Autodesk Inventor part; units mm, degrees
ref_plane "YZ Plane" through (0, 0, 0) normal (1, 0, 0) x (0, 1, 0)
ref_plane "XZ Plane" through (0, 0, 0) normal (0, 1, 0) x (-1, 0, 0)
ref_plane "XY Plane" through (0, 0, 0) normal (0, 0, 1) x (1, 0, 0)
sketch "스케치1" plane through (0, 0, 0) normal (0, 0, 1) x (1, 0, 0)
  line L0 (0, 0) -> (8.4524, -18.1262)
  line L1 (0, 0) -> (20, 0) construction
  line L2 (8.4524, -18.1262) -> (14.7965, -15.1678)
  line L3 (8.4524, -18.1262) -> (16.9047, -36.2523)
  line L4 (8.4524, -18.1262) -> (28.4524, -18.1262) construction
  arc A0 (16.9047, -36.2523) -> (0, 0) centre (-14.2701, -28.7218) ccw
  line L5 (0, 0) -> (0, 50)
  line L6 (0, 0) -> (50, 0) construction
  line L7 (0, 50) -> (12, 50)
  line L8 (12, 50) -> (12, 3)
  circle A1 centre (6, 44) radius 4.025
  circle A2 centre (6, 9) radius 4.025
  line L9 (16.9047, -36.2523) -> (26.8143, -31.6314)
  line L10 (16.9047, -36.2523) -> (27.8387, -36.2523) construction
  line L11 (12, -47.3039) -> (11.9482, -47.1928)
  arc A3 (26.2229, -36.2523) -> (12, 3) centre (-14.2701, -28.7218) ccw
  dimension "d16" = 20
  dimension "d17" = 65
  dimension "d18" = 7
  dimension "d19" = 90
  dimension "d20" = 20
  dimension "d21" = 65
  dimension "d22" = 50
  dimension "d23" = 90
  dimension "d24" = 12
  dimension "d25" = 90
  dimension "d26" = 47
  dimension "d27" = 8.05
  dimension "d28" = 8.05
  dimension "d29" = 6
  dimension "d30" = 6
  dimension "d31" = 6
  dimension "d32" = 35
  dimension "d33" = 25
extrude "돌출1" add sketch "스케치1" along normal blind 4 contours L5 L7 L8 A3 L9 A0
fillet "모깎기1" radius 6 2 edges at (12, 50, 2) (0, 50, 2)
sketch "스케치2" plane through (0, 0, 4) normal (0, 0, 1) x (1, 0, 0)
  line L0 (16.9047, -36.2523) -> (26.8143, -31.6314)
  arc A0 (17.3077, -34.3271) -> (18.715, -35.4082) centre (18.2923, -34.5019) ccw
  arc A1 (26.2765, -31.8822) -> (26.8523, -31.032) centre (25.8539, -30.9759) ccw
  line L1 (20, -34.809) -> (17.8869, -30.2774)
  line L2 (20, -34.809) -> (25, -34.809) construction
  line L3 (17.8869, -30.2774) -> (26.834, -26.1053)
  arc A2 (26.8143, -31.6314) -> (12, 3) centre (-14.2701, -28.7218) ccw
  line L4 (26.834, -26.1053) -> (17.7607, -30.3363)
  arc A3 (16.9047, -36.2523) -> (0, 0) centre (-14.2701, -28.7218) ccw
  arc A4 (26.2765, -31.8822) -> (26.8523, -31.032) centre (25.8539, -30.9759) ccw
  line L5 (26.834, -26.1053) -> (16.9047, -36.2523)
  line L6 (17.7607, -30.3363) -> (26.8143, -31.6314)
  circle A5 centre (22.0881, -30.9553) radius 1.6
  point P0 (12.3536, 2.7038)
  point P1 (0.5383, -0.2738)
  dimension "d38" = 5
  dimension "d39" = 115
  dimension "d40" = 90
  dimension "d41" = 3.2
extrude "돌출2" cut sketch "스케치2" against normal blind 4 contours A5 L6 L5 | L5 L6 A5 | A5 L5 L6 | L5 A5 L6
sketch "스케치4" plane through (0, 0, 4) normal (0, 0, 1) x (1, 0, 0)
  line L0 (12, 3) -> (12, 44)
  line L1 (12, 3) -> (2.5423, -1.4102)
  arc A0 (16.9047, -36.2523) -> (0, 0) centre (-14.2701, -28.7218) ccw
  line L2 (12, 3) -> (22.4355, 3) construction
  line L3 (7.2711, 0.7949) -> (9.8068, -4.643)
  line L4 (7.2711, 0.7949) -> (13.2711, 0.7949) construction
  line L5 (9.8068, -4.643) -> (7.8894, -5.5371)
  line L6 (9.8068, -4.643) -> (16.6121, -1.4696)
  arc A1 (26.8143, -31.6314) -> (12, 3) centre (-14.2701, -28.7218) ccw
  line L7 (9.8068, -4.643) -> (17.3156, -4.643) construction
  line L8 (2.5423, -1.4102) -> (16.6121, -1.4696)
  line L9 (7.8894, -5.5371) -> (12, 3)
  circle A2 centre (9.8616, -1.4411) radius 1.6
  dimension "d54" = 155
  dimension "d55" = 6
  dimension "d57" = 25
  dimension "d58" = 3.2
extrude "돌출4" cut sketch "스케치4" against normal up to surface (4 mm away) contours A2 L8 L9 | L9 L8 L3 A2 | L3 L8 A2 | A2 L9 L8 | L9 A2 L3 L8 | L8 L3 A2
sketch "스케치6" plane through (0, 0, 4) normal (0, 0, 1) x (1, 0, 0)
  line L0 (0, 0) -> (16.9047, -36.2523)
  circle A0 centre (9.8616, -1.4411) radius 1.6
  circle A1 centre (22.0881, -30.9553) radius 1.6
  arc A2 (12, 44) -> (0, 44) centre (6, 44) ccw
  line L1 (0, 44) -> (0, 0)
  arc A3 (16.9047, -36.2523) -> (0, 0) centre (-14.2701, -28.7218) ccw
  line L2 (16.9047, -36.2523) -> (26.8143, -31.6314)
  arc A4 (26.8143, -31.6314) -> (12, 3) centre (-14.2701, -28.7218) ccw
  line L3 (12, 3) -> (12, 44)
extrude "돌출6" add sketch "스케치6" against normal up to surface (4 mm away) contours A3 L0
fillet "모깎기3" radius 8 1 edges at (12, 3, 2)
properties part number "Grip_" material "알루미늄 6061"
Source: CAD feature listing. Evaluate the final solid. Frame: model axes, mm. A direction names the side the tool comes from. Round coordinates to 2 decimals unless told otherwise and drop trailing zeros. Loops run counter-clockwise (first coordinate to the right, second up) from the corner with the lowest first, then second, coordinate; pieces in that order, holes last. Notation, with made-up numbers: M 49.25,36.5 L 58.25,36.5 A15 ccw 58.25,55.5 Z; hole C -17.5,-15.75 d10. An arc over 180 degrees is marked long. Use a Markdown table: item, result. Add a question column.
1. Section query C-C on x = 22.75. Return the cut outline in (y, z), then the cut area to 3 significant figures.
2. Contact query for a flat-ended pin moving along its axis: P1, Ø2.5, axis at x = 22.09, y = -30.96, coming from the +Z side. Output: stop coordinate, or through.
3. Mould query, pull axis Y, two halves, no side actions, for faces 1 (the flat face through (10, 7, 4)), 2 (the cylindrical face through (5.13, 12.93, 1.97)), 3 (the flat face through (21.79, -33.974, 1.972)). Classes: pulls with the +Y half, pulls with the -Y half, needs draft (parallel to the pull), parting line crosses it, or undercut.
4. Section query D-D on y = 37. Return the cut outline in (x, z).
5. Section query A-A on y = 9. Return the cut outline in (x, z) (3 decimals), then the cut area to 3 significant figures.
6. Section query B-B on z = 1.6. Give the number of separate pieces and of enclosed holes in the cut face, then the cut area to 3 significant figures.
7. Line query: line 1 (Y direction, x = 6, z = 0.85) (3 decimals); line 2 (Y direction, x = 3, z = 1.75); line 3 (X direction, y = 39, z = 1). Output: solid intervals per line, ascending.
8. Reachability of faces 4 (the flat face through (12, 26, 2)), 5 (the cylindrical face through (9.5, -3, 2)) from +Z, -Z, +X, -X, +Y, -Y: full face, straight path, thin tool, end or side. Return the list, or none.
Reported:
| question | item | result |
|---|---|---|
| 1 | outline | M -33.53,0 L -32.41,0 L -32.41,4 L -33.53,4 Z; M -29.5,0 L -10.67,0 L -10.67,4 L -29.5,4 Z |
| 1 | area | 79.8 mm² |
| 2 | P1 | passes through |
| 3 | face 1 | needs draft |
| 3 | face 2 | undercut |
| 3 | face 3 | pulls with the -Y half |
| 4 | outline | M 0,0 L 12,0 L 12,4 L 0,4 Z |
| 5 | outline | M 0,0 L 1.975,0 L 1.975,4 L 0,4 Z; M 10.025,0 L 12,0 L 12,4 L 10.025,4 Z |
| 5 | area | 15.8 mm² |
| 6 | separate pieces | 1 |
| 6 | enclosed holes | 4 |
| 6 | area | 1,010 mm² |
| 7 | line 1 | y = -12.867 to 4.975, 13.025 to 39.975, 48.025 to 50 |
| 7 | line 2 | y = -6.43 to 6.32, 11.68 to 41.32, 46.68 to 49.2 |
| 7 | line 3 | x = 0 to 12 |
| 8 | face 4 | +Z, -Z, +X, +Y |
| 8 | face 5 | +Z, -Z |
